Could you check a few things on this model? Use its own coordinates, in mm. A direction names the side the tool comes from. Coordinates: 2 decimals unless noted, no trailing zeros. Loops run counter-clockwise (first coordinate to the right, second up) from the corner with the lowest first, then second, coordinate; pieces in that order, holes last. Notation, with made-up numbers: (19.25, -25) - (24.25, -25) arc R24 ccw to (24.25, -13) - close; hole circle Ø6 at (-21, -19.75). An arc over 180 degrees is marked (long way). One line per item, written item: value. Start each with the question number.
(1) If I drill on line 1 along Y through (x, z) = (80, 14.75); line 2 along Z through (x, y) = (114, 9), over which ranges is the centre line in solid material (lowest first)? Write a range as from..to.
(2) If we section it at B-B on x = 93.5: Write out the boundary of the cut face in (y, z).
(3) I'm going to push flat-ended pins straight in: P1, Ø7.5, axis at x = 103.5, y = 12, coming from the +Z side; P2, Ø6.5, axis at x = 115, z = 19.5, coming from the -Y side; P3, Ø6.5, axis at y = 15, z = 19.5, coming from the +X side. Where does each tip first touch, or does it pass through?
(4) On a 3-axis mill with a long thin cutter (end or side, diameter ignored), from which of +Z, -Z, +X, -X, +Y, -Y can I reach the whole of each face in a straight line? I mean faces 1 (the face through (75, 77, 0)), 2 (the face through (114, 25.4, 19)). Say none if no direction works.
(5) If we section it at A-A on z = 17.75: Write out the boundary of the cut face in (x, y), then the cut area to 3 significant figures.
```python
from build123d import *

# Parameters (mm, degrees)
F0_W       = 152.4
F0_H       = 152.4
F1_DEPTH   = 25.4
F2_W       = 76.2
F2_H       = 12.7
F1_FACE1_W = 152.4
F1_FACE1_H = 25.4
F3_DEPTH   = 25.4


with BuildPart() as f1:
    # F0 (on Top) → F1 (new body)
    with BuildSketch(Plane.XY):
        with Locations((76.2, 76.2)):
            Rectangle(F0_W, F0_H)
    extrude(amount=F1_DEPTH)

    # F2 (on face) + F1_face1 (on face) → F3 (cut)
    with BuildSketch(Plane.XZ):
        with Locations((114.3, 19.05)):
            Rectangle(F2_W, F2_H)
    with BuildSketch(Plane(origin=(76.2, 152.4, 12.7), x_dir=(-1, 0, 0), z_dir=(0, 1, 0))):
        Rectangle(F1_FACE1_W, F1_FACE1_H)
    extrude(amount=-F3_DEPTH, dir=(0, -1, 0), mode=Mode.SUBTRACT)


solid = f1.part
```
Values:
1. line 1: y = 25.4..152.4
1. line 2: z = 0..12.7
2. outline: (0, 0) - (152.4, 0) - (152.4, 25.4) - (25.4, 25.4) - (25.4, 12.7) - (0, 12.7) - close
3. P1: stops at z = 12.7
3. P2: stops at y = 25.4
3. P3: stops at x = 76.2
4. face 1: -Z, +X, -X, +Y, -Y
4. face 2: +Z, +X, -Y
5. outline: (0, 0) - (76.2, 0) - (76.2, 25.4) - (152.4, 25.4) - (152.4, 152.4) - (0, 152.4) - close
5. area: 21,300 mm2
